from build123d import *

# Parameters (mm, degrees)
Y_KSEKLIK_EKSTR_ZYON1_DEPTH = 1.5


with BuildPart() as part:
    # Çizim1 → Yükseklik-Ekstrüzyon1 (new body)
    with BuildSketch(Plane(origin=(0, 0, 0), x_dir=(1, 0, 0), z_dir=(0, 1, 0))):
        with BuildLine():
            Line((-20.9, -22.9), (20.9, -22.9))
            ThreePointArc((20.9, -22.9), (22.314213562, -22.314213562), (22.9, -20.9))
            Line((22.9, -20.9), (22.9, 20.9))
            ThreePointArc((22.9, 20.9), (22.314213562, 22.314213562), (20.9, 22.9))
            Line((20.9, 22.9), (-20.9, 22.9))
            ThreePointArc((-20.9, 22.9), (-22.314213562, 22.314213562), (-22.9, 20.9))
            Line((-22.9, 20.9), (-22.9, -20.9))
            ThreePointArc((-22.9, -20.9), (-22.314213562, -22.314213562), (-20.9, -22.9))
        make_face()
        with BuildLine():
            ThreePointArc((-2.705036995, 11.691140871), (0, -12), (2.705036995, 11.691140871))
            ThreePointArc((2.705036995, 11.691140871), (2.222647508, 11.958998982), (1.955748834, 12.441919973))
            ThreePointArc((1.955748834, 12.441919973), (0, 14), (-1.955748834, 12.441919973))
            ThreePointArc((-1.955748834, 12.441919973), (-2.222647508, 11.958998982), (-2.705036995, 11.691140871))
        make_face(mode=Mode.SUBTRACT)
    extrude(amount=Y_KSEKLIK_EKSTR_ZYON1_DEPTH)


solid = part.part
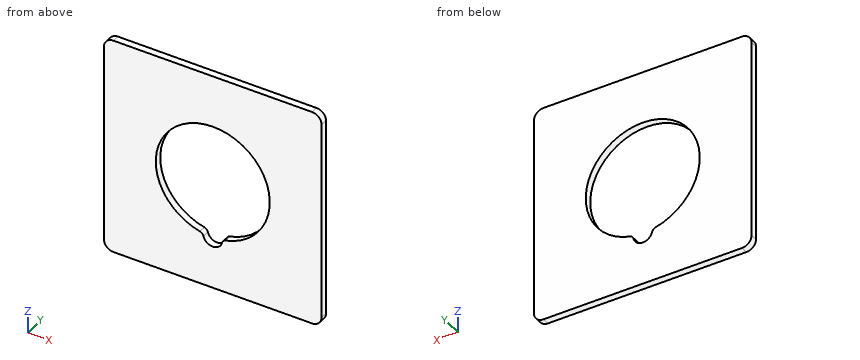
Geometry: final body of the model. Coordinates: model frame, mm. Give positions to 0.01 mm unless a question says otherwise; leave off trailing zeros. Write each loop counter-clockwise with the first axis right and the second up, starting at its lowest first coordinate (ties: lowest second). Pieces come first, ordered by that corner, then holes. Notation, with made-up numbers: M -22,26.25 L -2,26.25 A23 ccw -2,36.25 Z; hole C -5.5,13.25 d5. An arc over 180 degrees is marked long. Answer in a Markdown table with one row per item. Add a question column.
(1) Section B-B on z = 0. Return loops of the section in (x, y), and give its area (3 significant figures).
(2) Section A-A on y = 1. Return loops of the section in (x, z).
(3) Ray query, line 1 (X direction, y = 0.85, z = 0); line 2 (X direction, y = 1.25, z = -12.5); line 3 (X direction, y = 0.9, z = 21). Return the intervals inside material, ascending.
(4) Section C-C on x = 0. Return loops of the section in (y, z).
Result set:
| question | item | result |
|---|---|---|
| 1 | outline | M -22.9,0 L -12,0 L -12,1.5 L -22.9,1.5 Z; M 12,0 L 22.9,0 L 22.9,1.5 L 12,1.5 Z |
| 1 | area | 32.7 mm^2 |
| 2 | outline | M -22.9,-20.9 A2 ccw -20.9,-22.9 L 20.9,-22.9 A2 ccw 22.9,-20.9 L 22.9,20.9 A2 ccw 20.9,22.9 L -20.9,22.9 A2 ccw -22.9,20.9 Z; hole M -2.71,-11.69 A1 cw -1.96,-12.44 A2.01 ccw 1.96,-12.44 A1 cw 2.71,-11.69 A12 ccw long Z |
| 3 | line 1 | x = -22.9 to -12, 12 to 22.9 |
| 3 | line 2 | x = -22.9 to -1.94, 1.94 to 22.9 |
| 3 | line 3 | x = -22.9 to 22.9 |
| 4 | outline | M 0,-22.9 L 1.5,-22.9 L 1.5,-14 L 0,-14 Z; M 0,12 L 1.5,12 L 1.5,22.9 L 0,22.9 Z |
